from build123d import *

# Parameters (mm, degrees)
F0_W     = 400
F0_H     = 150
F0_W_2   = 14.666667
F0_H_2   = 3.175
F0_R     = 1.64084
F0_W_3   = 12.7
F0_W_4   = 3.175
F0_H_3   = 5.08
F0_H_4   = 3.215846
F0_R_2   = 3.302
F1_DEPTH = 3.175


with BuildPart() as f1:
    # F0 (on Front) → F1 (new body)
    with BuildSketch(Plane.XZ):
        Rectangle(F0_W, F0_H)
        with Locations((-101.366666, -69.285)):
            Rectangle(F0_W_2, F0_H_2, mode=Mode.SUBTRACT)
        with Locations((-150.9747, -52.45)):
            Circle(F0_R, mode=Mode.SUBTRACT)
        with Locations((-124.0253, -52.45)):
            Circle(F0_R, mode=Mode.SUBTRACT)
        with Locations((-72.033333, -69.285)):
            Rectangle(F0_W_2, F0_H_2, mode=Mode.SUBTRACT)
        with Locations((-130.175, -25.590497)):
            Rectangle(F0_W_3, F0_H_2, mode=Mode.SUBTRACT)
        with Locations((-104.775, -25.590497)):
            Rectangle(F0_W_3, F0_H_2, mode=Mode.SUBTRACT)
        with Locations((-157.1625, -10.032997)):
            Rectangle(F0_W_4, F0_H_3, mode=Mode.SUBTRACT)
        with Locations((-79.375, -25.590497)):
            Rectangle(F0_W_3, F0_H_2, mode=Mode.SUBTRACT)
        with Locations((-53.975, -25.590497)):
            Rectangle(F0_W_3, F0_H_2, mode=Mode.SUBTRACT)
        with Locations((-28.575, -25.590497)):
            Rectangle(F0_W_3, F0_H_2, mode=Mode.SUBTRACT)
        with Locations((-1.5875, -10.032997)):
            Rectangle(F0_W_4, F0_H_3, mode=Mode.SUBTRACT)
        with Locations((124.0253, -52.45)):
            Circle(F0_R, mode=Mode.SUBTRACT)
        with Locations((150.9747, -52.45)):
            Circle(F0_R, mode=Mode.SUBTRACT)
        with Locations((86.7, -12.720423)):
            Rectangle(F0_W_3, F0_H_4, mode=Mode.SUBTRACT)
        with Locations((112.1, -12.720423)):
            Rectangle(F0_W_3, F0_H_4, mode=Mode.SUBTRACT)
        with Locations((-157.1625, 0.127003)):
            Rectangle(F0_W_4, F0_H_3, mode=Mode.SUBTRACT)
        with Locations((-157.1625, 10.287003)):
            Rectangle(F0_W_4, F0_H_3, mode=Mode.SUBTRACT)
        with Locations((-130.175, 25.844503)):
            Rectangle(F0_W_3, F0_H_2, mode=Mode.SUBTRACT)
        with Locations((-104.775, 25.844503)):
            Rectangle(F0_W_3, F0_H_2, mode=Mode.SUBTRACT)
        with Locations((-1.5875, 0.127003)):
            Rectangle(F0_W_4, F0_H_3, mode=Mode.SUBTRACT)
        with Locations((-1.5875, 10.287003)):
            Rectangle(F0_W_4, F0_H_3, mode=Mode.SUBTRACT)
        with Locations((-79.375, 25.844503)):
            Rectangle(F0_W_3, F0_H_2, mode=Mode.SUBTRACT)
        with Locations((-53.975, 25.844503)):
            Rectangle(F0_W_3, F0_H_2, mode=Mode.SUBTRACT)
        with Locations((-28.575, 25.844503)):
            Rectangle(F0_W_3, F0_H_2, mode=Mode.SUBTRACT)
        with Locations((-150.9747, 52.45)):
            Circle(F0_R, mode=Mode.SUBTRACT)
        with Locations((-124.0253, 52.45)):
            Circle(F0_R, mode=Mode.SUBTRACT)
        with Locations((-101.366666, 69.285)):
            Rectangle(F0_W_2, F0_H_2, mode=Mode.SUBTRACT)
        with Locations((-72.033333, 69.285)):
            Rectangle(F0_W_2, F0_H_2, mode=Mode.SUBTRACT)
        Polygon((156.55, 7.9375), (156.55, -7.9375), (118.45, -7.9375), (80.35, -7.9375), (67.65, -7.9375), (67.65, 7.9375), (80.35, 7.9375), (118.45, 7.9375), align=None, mode=Mode.SUBTRACT)
        with Locations((177.14, 0)):
            Circle(F0_R_2, mode=Mode.SUBTRACT)
        with Locations((124.0253, 52.45)):
            Circle(F0_R, mode=Mode.SUBTRACT)
        with Locations((150.9747, 52.45)):
            Circle(F0_R, mode=Mode.SUBTRACT)
    extrude(amount=F1_DEPTH)


solid = f1.part
For this review, take the finished solid that the model builds, in its own axes (mm). Coordinates: 2 decimals unless noted, no trailing zeros. Order: outer loops, then holes, each group sorted by start corner. A loop starts at its lowest first (then second) coordinate and runs counter-clockwise, first axis right, second up. Notation, with made-up numbers: (26, -34.5) - (63, -34.5) arc R26 cw to (63, -15.5) - close; hole circle Ø10 at (-37.75, 36.25). An arc over 180 degrees is marked (long way). Answer as CSV lines item,"result". Start each with the question number.
1) Draft analysis for pull direction X (two halves, no side actions). For faces 1 (the cylindrical face through (173.84, -1.57, 0.15)), 2 (the flat face through (-3, 0, 18)), state which applies: +X half, -X half, draft (parallel to the pull), parting line (faces both ways), or undercut.
2) Add section B-B (y = -0.8). Count the separate pieces of the cut face and the enclosed holes in it, then the cut area to 3 significant figures.
3) Add section A-A (x = 134). State the section outline as (y, z) points (1 decimal).
4) To check wall thickness, follow line 1 along Z through (x, y) = (87, -0.2); line 2 along X through (y, z) = (-1.65, 2) (3 decimals); line 3 along Z through (x, y) = (177.14, -2.45). State the ranges of each line that lie inside material, in increasing order. Write a range as [from, to].
Result:
1,face 1,"undercut"
1,face 2,"draft"
2,separate pieces,"1"
2,enclosed holes,"32"
2,area,"57,700 mm^2"
3,outline,"(-3.2, -75) - (0, -75) - (0, -7.9) - (-3.2, -7.9) - close; (-3.2, 7.9) - (0, 7.9) - (0, 75) - (-3.2, 75) - close"
4,line 1,"[-75, -14.33], [-11.11, -7.94], [7.94, 75]"
4,line 2,"[-200, -158.75], [-155.575, -3.175], [0, 67.65], [156.55, 174.513], [179.767, 200]"
4,line 3,"[-75, -3.3], [3.3, 75]"
